from build123d import *

# Parameters (mm, degrees)
SKETCH1_W           = 56
SKETCH1_H           = 33
BOSS_EXTRUDE1_DEPTH = 0.5
SKETCH2_W           = 27
SKETCH2_H           = 16.5
CUT_EXTRUDE1_DEPTH  = 0.5
SKETCH3_R           = 4.7
BOSS_EXTRUDE2_DEPTH = 1
FILLET1_R           = 1
SKETCH4_W           = 2.5
SKETCH4_H           = 16
BOSS_EXTRUDE3_DEPTH = 15
FILLET2_R           = 3


with BuildPart() as part:
    # Sketch1 → Boss-Extrude1 (new body)
    with BuildSketch(Plane.XY):
        Rectangle(SKETCH1_W, SKETCH1_H)
    extrude(amount=BOSS_EXTRUDE1_DEPTH)

    # Sketch2 → Cut-Extrude1 (cut)
    with BuildSketch(Plane.XY.offset(0.5)):
        with Locations((-4.5, 3.75)):
            Rectangle(SKETCH2_W, SKETCH2_H)
    extrude(amount=-CUT_EXTRUDE1_DEPTH, mode=Mode.SUBTRACT)

    # Sketch3 → Boss-Extrude2 (add)
    with BuildSketch(Plane.XY.offset(0.5)):
        with Locations((-13.8, -10.75)):
            Circle(SKETCH3_R)
        with Locations((4.8, -10.75)):
            Circle(SKETCH3_R)
    extrude(amount=BOSS_EXTRUDE2_DEPTH)

    # Fillet1
    fillet1_edges = [part.edges().sort_by_distance(p)[0] for p in [
        (-18.5, -10.75, 1.5),
        (0.1, -10.75, 1.5),
    ]]
    fillet(fillet1_edges, radius=FILLET1_R - 0.0001)  # a hair under: the kernel refuses the full size

    # Sketch4 → Boss-Extrude3 (add)
    with BuildSketch(Plane(origin=(0, 0, 0), x_dir=(-1, 0, 0), z_dir=(0, 0, -1))):
        with Locations((-24.25, -0.75)):
            Rectangle(SKETCH4_W, SKETCH4_H)
    extrude(amount=BOSS_EXTRUDE3_DEPTH)

    # Fillet2
    fillet2_edges = [part.edges().sort_by_distance(p)[0] for p in [
        (28, -16.5, 0.25),
        (-28, -16.5, 0.25),
        (-28, 16.5, 0.25),
        (28, 16.5, 0.25),
    ]]
    fillet(fillet2_edges, radius=FILLET2_R)


solid = part.part
Geometry: final body of the model. Coordinates: model frame, mm. A direction names the side the tool comes from. Give positions to 0.01 mm unless a question says otherwise; leave off trailing zeros. Write each loop counter-clockwise with the first axis right and the second up, starting at its lowest first coordinate (ties: lowest second). Pieces come first, ordered by that corner, then holes.
(1) Mould query, pull axis X, two halves, no side actions, for faces 6 (the cylindrical face through (27.1, -15.64, 0.25)), 7 (the flat face through (0, -7, 0)), 8 (the flat face through (23, -1, -7)). Classes: released by +X, released by -X, zero draft, split by the parting line, or undercut.
(2) Cut plane D-D, the plane z = -12.5. Return loops of the section in (x, y).
(3) Cut plane A-A, the plane x = -1. Return loops of the section in (y, z).
(4) Access query for faces 1 (the flat face through (25.5, -1, -7)), 2 (the flat face through (-14, -11, 1.5)), 3 (the flat face through (24, 7.25, -7)), 4 (the flat face through (24, -8.75, -7)), 5 (the cylindrical face through (-27.14, -15.6, 0.25)). Directions: +Z, -Z, +X, -X, +Y, -Y. A direction counts if a zero-diameter tool reaches every point of the face in a straight line with its end or side. Return the directions, or none.
(5) Ray query, line 1 (Z direction, x = 17.5, y = -11.5); line 2 (X direction, y = 6.5, z = -13); line 3 (Z direction, x = 23.5, y = -2). Return the intervals inside material, ascending.
(6) First-contact query: P1, Ø12, axis at x = 8, y = -2, coming from the -Z side; P2, Ø0.8, axis at x = 23.5, z = -8, coming from the -Y side; P3, Ø8, axis at y = -4.5, z = -9, coming from the +X side. Flat tips, straight axial feed; report the tip coordinate or a pass-through.
Values follow:
1. face 6: released by +X
1. face 7: zero draft
1. face 8: released by -X
2. outline: (23, -8.75) - (25.5, -8.75) - (25.5, 7.25) - (23, 7.25) - close
3. outline: (-16.5, 0) - (-4.5, 0) - (-4.5, 0.5) - (-16.5, 0.5) - close; (12, 0) - (16.5, 0) - (16.5, 0.5) - (12, 0.5) - close
4. face 1: -Z, +X, +Y, -Y
4. face 2: +Z, +X, -X, +Y, -Y
4. face 3: -Z, +X, -X, +Y
4. face 4: -Z, +X, -X, -Y
4. face 5: +Z, -Z, -X, -Y
5. line 1: z = 0 to 0.5
5. line 2: x = 23 to 25.5
5. line 3: z = -15 to 0.5
6. P1: stops at z = 0
6. P2: stops at y = -8.75
6. P3: stops at x = 25.5
